Part model, mm, in its own coordinate system. A direction names the side the tool comes from. Give positions to 0.01 mm unless a question says otherwise; leave off trailing zeros. Order: outer loops, then holes, each group sorted by start corner. A loop starts at its lowest first (then second) coordinate and runs counter-clockwise, first axis right, second up. Notation, with made-up numbers: (53.5, 57.25) - (107.5, 57.25) arc R23 cw to (107.5, 65.25) - close; hole circle Ø3 at (-5.5, -8.75). An arc over 180 degrees is marked (long way). One line per item, written item: value.
```python
from build123d import *

# Parameters (mm, degrees)
BOSS_EXTRUDE1_DEPTH = 4
BOSS_EXTRUDE3_DEPTH = 4
SKETCH6_R           = 2
CUT_EXTRUDE1_DEPTH  = 18
BOSS_EXTRUDE4_DEPTH = 18
SKETCH8_R           = 2.25
CUT_EXTRUDE2_DEPTH  = 68.060778195
SKETCH10_W          = 25.230248524
SKETCH10_H          = 17.693033904
CUT_EXTRUDE4_DEPTH  = 66.862040733


with BuildPart() as part:
    # Sketch2 → Boss-Extrude1 (new body)
    with BuildSketch(Plane.XY):
        with BuildLine():
            Line((17.593003447, 3.447921134), (18.432689254, 3.812129579))
            ThreePointArc((18.432689254, 3.812129579), (18.142308848, 4.822341152), (17.760116965, 5.801513031))
            Line((17.760116965, 5.801513031), (16.871688472, 5.581479263))
            Line((16.871688472, 5.581479263), (15.649099733, 5.241598415))
            ThreePointArc((15.649099733, 5.241598415), (15.22663553, 6.009376293), (14.733410626, 6.733729845))
            Line((14.733410626, 6.733729845), (15.590096731, 7.669855443))
            Line((15.590096731, 7.669855443), (16.188603379, 8.362321932))
            ThreePointArc((16.188603379, 8.362321932), (15.488665299, 9.146499772), (14.719475556, 9.862876308))
            Line((14.719475556, 9.862876308), (14.014498216, 9.279158058))
            Line((14.014498216, 9.279158058), (13.060452596, 8.442474621))
            ThreePointArc((13.060452596, 8.442474621), (12.346699165, 8.950918239), (11.588033655, 9.389535972))
            Line((11.588033655, 9.389535972), (11.95371149, 10.604658163))
            Line((11.95371149, 10.604658163), (12.192497398, 11.488231214))
            ThreePointArc((12.192497398, 11.488231214), (11.221632964, 11.891059284), (10.217792822, 12.202753318))
            Line((10.217792822, 12.202753318), (9.835896044, 11.370963143))
            Line((9.835896044, 11.370963143), (9.33935398, 10.203192533))
            ThreePointArc((9.33935398, 10.203192533), (8.475678941, 10.351598396), (7.601835833, 10.417606691))
            Line((7.601835833, 10.417606691), (7.404078418, 11.671055622))
            Line((7.404078418, 11.671055622), (7.235849109, 12.570732756))
            ThreePointArc((7.235849109, 12.570732756), (6.18634993, 12.512426015), (5.14668224, 12.357702722))
            Line((5.14668224, 12.357702722), (5.163505363, 11.442586867))
            Line((5.163505363, 11.442586867), (5.222813101, 10.175020376))
            ThreePointArc((5.222813101, 10.175020376), (4.380277888, 9.933994883), (3.564332526, 9.614319987))
            Line((3.564332526, 9.614319987), (2.842308143, 10.657834724))
            Line((2.842308143, 10.657834724), (2.300383494, 11.395423851))
            ThreePointArc((2.300383494, 11.395423851), (1.380115753, 10.887530665), (0.510539453, 10.297034891))
            Line((0.510539453, 10.297034891), (0.922750452, 9.479843274))
            Line((0.922750452, 9.479843274), (1.526161366, 8.363537991))
            ThreePointArc((1.526161366, 8.363537991), (0.871640411, 7.780819197), (0.275200782, 7.138776643))
            Line((0.275200782, 7.138776643), (-0.828084785, 7.765676295))
            Line((-0.828084785, 7.765676295), (-1.636369952, 8.195088843))
            ThreePointArc((-1.636369952, 8.195088843), (-2.245135941, 7.338203686), (-2.772390602, 6.42889036))
            Line((-2.772390602, 6.42889036), (-2.04643517, 5.871477804))
            Line((-2.04643517, 5.871477804), (-1.018434012, 5.12753168))
            ThreePointArc((-1.018434012, 5.12753168), (-1.355304806, 4.318534189), (-1.61410652, 3.481288379))
            Line((-1.61410652, 3.481288379), (-2.880134034, 3.567407782))
            Line((-2.880134034, 3.567407782), (-3.794688927, 3.603593329))
            ThreePointArc((-3.794688927, 3.603593329), (-3.971379595, 2.567432815), (-4.051883364, 1.519402593))
            Line((-4.051883364, 1.519402593), (-3.155967876, 1.332171491))
            Line((-3.155967876, 1.332171491), (-1.90698471, 1.107932181))
            ThreePointArc((-1.90698471, 1.107932181), (-1.859483953, 0.232887867), (-1.729388897, -0.633734398))
            Line((-1.729388897, -0.633734398), (-2.907406081, -1.105452248))
            Line((-2.907406081, -1.105452248), (-3.747091888, -1.469660694))
            ThreePointArc((-3.747091888, -1.469660694), (-3.456711482, -2.479872267), (-3.0745196, -3.459044145))
            Line((-3.0745196, -3.459044145), (-2.186091107, -3.239010378))
            Line((-2.186091107, -3.239010378), (-0.963502367, -2.899129529))
            ThreePointArc((-0.963502367, -2.899129529), (-0.541038164, -3.666907408), (-0.047813261, -4.391260959))
            Line((-0.047813261, -4.391260959), (-0.904499365, -5.327386558))
            Line((-0.904499365, -5.327386558), (-1.503006014, -6.019853046))
            ThreePointArc((-1.503006014, -6.019853046), (-0.803067933, -6.804030887), (-0.03387819, -7.520407423))
            Line((-0.03387819, -7.520407423), (0.67109915, -6.936689172))
            Line((0.67109915, -6.936689172), (1.625144769, -6.100005735))
            ThreePointArc((1.625144769, -6.100005735), (2.3388982, -6.608449353), (3.097563711, -7.047067087))
            Line((3.097563711, -7.047067087), (2.731885876, -8.262189278))
            Line((2.731885876, -8.262189278), (2.493099968, -9.145762328))
            ThreePointArc((2.493099968, -9.145762328), (3.463964401, -9.548590398), (4.467804544, -9.860284433))
            Line((4.467804544, -9.860284433), (4.849701322, -9.028494257))
            Line((4.849701322, -9.028494257), (5.346243386, -7.860723648))
            ThreePointArc((5.346243386, -7.860723648), (6.209918425, -8.009129511), (7.083761533, -8.075137806))
            Line((7.083761533, -8.075137806), (7.281518948, -9.328586736))
            Line((7.281518948, -9.328586736), (7.449748257, -10.22826387))
            ThreePointArc((7.449748257, -10.22826387), (8.499247436, -10.16995713), (9.538915126, -10.015233837))
            Line((9.538915126, -10.015233837), (9.522092003, -9.100117982))
            Line((9.522092003, -9.100117982), (9.462784265, -7.83255149))
            ThreePointArc((9.462784265, -7.83255149), (10.305319478, -7.591525998), (11.12126484, -7.271851101))
            Line((11.12126484, -7.271851101), (11.843289223, -8.315365839))
            Line((11.843289223, -8.315365839), (12.385213872, -9.052954966))
            ThreePointArc((12.385213872, -9.052954966), (13.305481612, -8.54506178), (14.175057913, -7.954566005))
            Line((14.175057913, -7.954566005), (13.762846914, -7.137374389))
            Line((13.762846914, -7.137374389), (13.159436, -6.021069105))
            ThreePointArc((13.159436, -6.021069105), (13.813956955, -5.438350311), (14.410396584, -4.796307757))
            Line((14.410396584, -4.796307757), (15.513682151, -5.42320741))
            Line((15.513682151, -5.42320741), (16.321967317, -5.852619957))
            ThreePointArc((16.321967317, -5.852619957), (16.930733307, -4.9957348), (17.457987967, -4.086421474))
            Line((17.457987967, -4.086421474), (16.732032536, -3.529008918))
            Line((16.732032536, -3.529008918), (15.704031377, -2.785062794))
            ThreePointArc((15.704031377, -2.785062794), (16.040902172, -1.976065303), (16.299703886, -1.138819493))
            Line((16.299703886, -1.138819493), (17.565731399, -1.224938896))
            Line((17.565731399, -1.224938896), (18.480286292, -1.261124443))
            ThreePointArc((18.480286292, -1.261124443), (18.656976961, -0.22496393), (18.737480729, 0.823066292))
            Line((18.737480729, 0.823066292), (17.841565242, 1.010297394))
            Line((17.841565242, 1.010297394), (16.592582076, 1.234536705))
            ThreePointArc((16.592582076, 1.234536705), (16.545081318, 2.109581019), (16.414986263, 2.976203284))
            Line((16.414986263, 2.976203284), (17.593003447, 3.447921134))
        make_face()
    extrude(amount=-BOSS_EXTRUDE1_DEPTH)

    # Sketch5 → Boss-Extrude3 (add)
    with BuildSketch(Plane.XY):
        with BuildLine():
            Line((34.627961915, -50.407866333), (38.369192873, -48.55177457))
            Line((38.369192873, -48.55177457), (13.393984011, -14.920355903))
            Line((13.393984011, -14.920355903), (9.462784265, -7.83255149))
            Line((9.462784265, -7.83255149), (0.865656202, -2.843190202))
            Line((0.865656202, -2.843190202), (-0.03387819, -7.520407423))
            add(Edge.make_bspline(
                [(34.627961915, -50.407866333), (20.737528927, -38.343464696), (7.957182105, -24.264537371), (-0.03387819, -7.520407423)],
                knots=[0, 0, 0, 0, 1, 1, 1, 1], degree=3))
        make_face()
    extrude(amount=-BOSS_EXTRUDE3_DEPTH)

    # Sketch6 → Cut-Extrude1 (cut)
    with BuildSketch(Plane(origin=(0, 0, -4), x_dir=(-1, 0, 0), z_dir=(0, 0, -1))):
        with Locations((-7.342798683, 1.171234443)):
            Circle(SKETCH6_R)
    extrude(amount=-CUT_EXTRUDE1_DEPTH, mode=Mode.SUBTRACT)

    # Sketch7 → Boss-Extrude4 (add)
    with BuildSketch(Plane.XY):
        with BuildLine():
            Line((34.627961915, -50.407866333), (38.369192873, -48.55177457))
            Line((38.369192873, -48.55177457), (13.393984011, -14.920355903))
            add(Edge.make_bspline(
                [(7.977955023, -21.345123668), (8.112113434, -15.921271934), (13.393984011, -14.920355903)],
                knots=[0, 0, 0, 1, 1, 1], degree=2))
            add(Edge.make_bspline(
                [(7.977955023, -21.345123668), (15.413845314, -32.210109704), (24.739621619, -41.819443715), (34.627961915, -50.407866333)],
                knots=[0.288118642, 0.288118642, 0.288118642, 0.288118642, 1, 1, 1, 1], degree=3))
        make_face()
    extrude(amount=BOSS_EXTRUDE4_DEPTH)

    # Sketch8 → Cut-Extrude2 (cut, through all)
    with BuildSketch(Plane(origin=(0, 0, -4), x_dir=(-1, 0, 0), z_dir=(0, 0, -1))):
        with Locations((-16.490179828, -25.746560684)):
            Circle(SKETCH8_R)
        with Locations((-25.785580409, -37.215397344)):
            Circle(SKETCH8_R)
    extrude(amount=-CUT_EXTRUDE2_DEPTH, mode=Mode.SUBTRACT)

    # Sketch10 → Cut-Extrude4 (cut, through all)
    with BuildSketch(Plane(origin=(1.491415785, 1.107548305, 0), x_dir=(0, 0, -1), z_dir=(0.8028367498889462, 0.5961989206865052, 0))):
        with Locations((-14.573721534, -16.286562524)):
            Rectangle(SKETCH10_W, SKETCH10_H)
    extrude(amount=-CUT_EXTRUDE4_DEPTH, mode=Mode.SUBTRACT)


solid = part.part
```
1) Two-plate mould, pull along Y, no slides. Class faces 4 (the face through (7.504, 11.036, -1.972)), 5 (the face through (-0.547, -3.656, -1.972)), 6 (the face through (11, -19, 1.959)): pulls with the +Y half, pulls with the -Y half, needs draft (parallel to the pull), parting line crosses it, or undercut.
Answer:
face 4: pulls with the +Y half
face 5: undercut
face 6: needs draft
2) Drop flat-ended pins along their axis: P1, Ø8, axis at x = 6, y = -14.5, coming from the +Z side; P2, Ø3, axis at x = 19.5, z = 12, coming from the +Y side; P3, Ø9.5, axis at x = 10.5, y = -17.5, coming from the +Z side. Give the stop position or say it passes through.
Answer:
P1: stops at z = 0
P2: stops at y = -21.12
P3: stops at z = 1.96
3) Wall check: line 1 along X through (y, z) = (-5, -1.5); line 2 along Z through (x, y) = (0, 5); line 3 along X through (y, z) = (-39, 9.5). Give the ranges that are in metal, low to high. Write a range as [from, to].
Answer:
line 1: x = [-0.6, 14.23], [14.77, 16.93]
line 2: z = [-4, 0]
line 3: x = [22.54, 24.42], [27.16, 31.28]
4) Slice it at A-A on y = 0. Write the cut outline in (x, z).
Answer:
outline: (-1.83, -4) - (5.72, -4) - (5.72, 0) - (-1.83, 0) - close; (8.96, -4) - (18.68, -4) - (18.68, 0) - (8.96, 0) - close
5) Slice it at B-B on z = -1. Count the separate pieces of the cut face and the enclosed holes in it, then the cut area to 3 significant figures.
Answer:
separate pieces: 1
enclosed holes: 3
area: 668 mm2
6) Which spindle directions (+Z, -Z, +X, -X, +Y, -Y) get a long thin tool onto all of the face, cutting with end or side? Do faces 1 (the face through (5.193, 10.818, -1.972)), 2 (the face through (17.23, 1.12, -1.97)), 3 (the face through (13.207, -21.498, 10.092)). Say none if no direction does.
Answer:
face 1: +Z, -Z
face 2: +Z, -Z, +X
face 3: +Z, -X, +Y
